Check sheet for the modelled part. Datum: model origin and axes. Units: mm. Coordinates: 2 decimals unless noted, no trailing zeros. Loops run counter-clockwise (first coordinate to the right, second up) from the corner with the lowest first, then second, coordinate; pieces in that order, holes last. Notation, with made-up numbers: (86, -3) -> (126, -3) arc R25 cw to (126, 25) -> close; hole circle Ø10 at (7, 85.25). An arc over 180 degrees is marked (long way). Use one line per item in the form item = value.
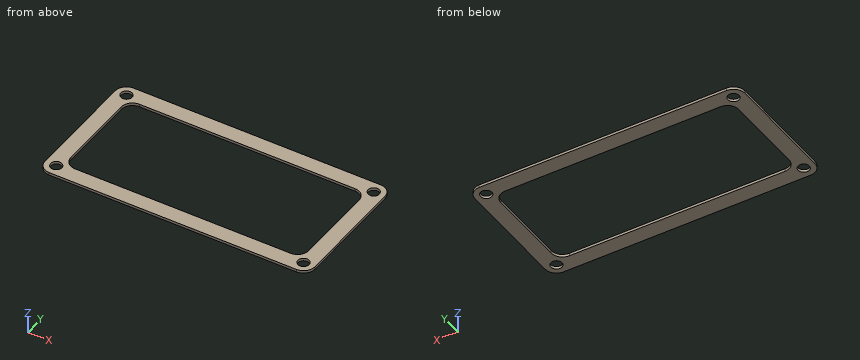
from build123d import *

# Parameters (mm, degrees)
F1_DEPTH = 6
F2_D     = 25
F3_D     = 25
F4_D     = 25


with BuildPart() as f1:
    # F0 (on Top) → F1 (new body)
    with BuildSketch(Plane.XY):
        with BuildLine():
            Line((-275, -150), (275, -150))
            ThreePointArc((275, -150), (292.67767, -142.67767), (300, -125))
            Line((300, -125), (300, 125))
            ThreePointArc((300, 125), (292.67767, 142.67767), (275, 150))
            Line((275, 150), (-275, 150))
            ThreePointArc((-275, 150), (-292.67767, 142.67767), (-300, 125))
            Line((-300, 125), (-300, -125))
            ThreePointArc((-300, -125), (-292.67767, -142.67767), (-275, -150))
        make_face()
        with BuildLine():
            ThreePointArc((264.644661, -89.644661), (257.32233, -107.32233), (239.644661, -114.644661))
            Line((239.644661, -114.644661), (-239.644661, -114.644661))
            ThreePointArc((-239.644661, -114.644661), (-257.32233, -107.32233), (-264.644661, -89.644661))
            Line((-264.644661, -89.644661), (-264.644661, 89.644661))
            ThreePointArc((-264.644661, 89.644661), (-257.32233, 107.32233), (-239.644661, 114.644661))
            Line((-239.644661, 114.644661), (239.644661, 114.644661))
            ThreePointArc((239.644661, 114.644661), (257.32233, 107.32233), (264.644661, 89.644661))
            Line((264.644661, 89.644661), (264.644661, -89.644661))
        make_face(mode=Mode.SUBTRACT)
    extrude(amount=F1_DEPTH)

    # F2 (through all)
    with Locations(Plane(origin=(0, 0, 0), x_dir=(1, 0, 0), z_dir=(0, 0, -1))):
        with Locations((-275, -125)):
            Hole(F2_D / 2)

    # F3 (through all)
    with Locations(Plane(origin=(0, 0, 0), x_dir=(1, 0, 0), z_dir=(0, 0, -1))):
        with Locations((-275, 125), (275, -125)):
            Hole(F3_D / 2)

    # F4 (through all)
    with Locations(Plane(origin=(0, 0, 0), x_dir=(1, 0, 0), z_dir=(0, 0, -1))):
        with Locations((275, 125)):
            Hole(F4_D / 2)


solid = f1.part
(1) Section check B-B, the plane x = -170. Record the boundary of the cut face in (y, z).
Established:
outline = (-150, 0) -> (-114.64, 0) -> (-114.64, 6) -> (-150, 6) -> close; (114.64, 0) -> (150, 0) -> (150, 6) -> (114.64, 6) -> close
(2) Section check A-A, the plane y = -77. Record the boundary of the cut face in (x, z), plus the area to 3 significant figures.
Established:
outline = (-300, 0) -> (-264.64, 0) -> (-264.64, 6) -> (-300, 6) -> close; (264.64, 0) -> (300, 0) -> (300, 6) -> (264.64, 6) -> close
area = 424 mm²
(3) Section check C-C, the plane z = 1.75. Record the boundary of the cut face in (x, y), plus the area to 3 significant figures.
Established:
outline = (-300, -125) arc R25 ccw to (-275, -150) -> (275, -150) arc R25 ccw to (300, -125) -> (300, 125) arc R25 ccw to (275, 150) -> (-275, 150) arc R25 ccw to (-300, 125) -> close; hole circle Ø25 at (-275, -125); hole circle Ø25 at (-275, 125); hole (-264.64, -89.64) arc R25 ccw to (-239.64, -114.64) -> (239.64, -114.64) arc R25 ccw to (264.64, -89.64) -> (264.64, 89.64) arc R25 ccw to (239.64, 114.64) -> (-239.64, 114.64) arc R25 ccw to (-264.64, 89.64) -> close; hole circle Ø25 at (275, -125); hole circle Ø25 at (275, 125)
area = 56,700 mm²
(4) Scan lines: line 1 along Y through (x, z) = (-275, 2); line 2 along X through (y, z) = (125, 3.25); line 3 along X through (y, z) = (-74, 3.05). Record each from-to range of solid material in increasing order.
Established:
line_1 = -150 to -137.5, -112.5 to 112.5, 137.5 to 150
line_2 = -300 to -287.5, -262.5 to 262.5, 287.5 to 300
line_3 = -300 to -264.64, 264.64 to 300
